from build123d import *

# Parameters (mm, degrees)
SKETCH090_W     = 20
SKETCH090_H     = 10
PAD049_DEPTH    = 10
SKETCH091_W     = 20
SKETCH091_H     = 6
PAD050_DEPTH    = 15
SKETCH092_W     = 1.5
SKETCH092_H     = 15
PAD051_DEPTH    = 0.9
SKETCH093_W     = 17
SKETCH093_H     = 3.5
POCKET033_DEPTH = 16
SKETCH094_W     = 0.8
SKETCH094_H     = 0.3
POCKET034_DEPTH = 20
SKETCH095_W     = 0.8
SKETCH095_H     = 0.3
POCKET035_DEPTH = 20
SKETCH006_W     = 18
SKETCH006_H     = 8
POCKET003_DEPTH = 8
SKETCH096_W     = 0.8
SKETCH096_H     = 0.7
POCKET036_DEPTH = 2
SKETCH097_W     = 0.8
SKETCH097_H     = 0.5
POCKET037_DEPTH = 5
FILLET_R        = 0.17
CHAMFER054_SIZE = 0.3
CHAMFER007_SIZE = 0.3
FILLET001_R     = 0.15


with BuildPart() as part:
    # Sketch090 → Pad049 (new body)
    with BuildSketch(Plane.XZ):
        Rectangle(SKETCH090_W, SKETCH090_H)
    extrude(amount=-PAD049_DEPTH)

    # Sketch091 (on Face5 of Pad049) → Pad050 (join)
    with BuildSketch(Plane.XZ):
        Rectangle(SKETCH091_W, SKETCH091_H)
    extrude(amount=PAD050_DEPTH)

    # Sketch092 (on Face7 of Pad050) → Pad051 (join)
    with BuildSketch(Plane(origin=(0, 0, -3), x_dir=(1, 0, 0), z_dir=(0, 0, -1))):
        with Locations((-7.25, 7.5)):
            Rectangle(SKETCH092_W, SKETCH092_H)
        with Locations((7.25, 7.5)):
            Rectangle(SKETCH092_W, SKETCH092_H)
    extrude(amount=PAD051_DEPTH)

    # Sketch093 (on Face18 of Pad051) → Pocket033 (cut)
    with BuildSketch(Plane.XZ.offset(15)):
        with Locations((0, -0.25)):
            Rectangle(SKETCH093_W, SKETCH093_H)
    extrude(amount=-POCKET033_DEPTH, mode=Mode.SUBTRACT)

    # Sketch094 (on Face9 of Pocket033) → Pocket034 (cut)
    with BuildSketch(Plane.XZ.offset(15)):
        with Locations((-3.4, -2.15)):
            Rectangle(SKETCH094_W, SKETCH094_H)
        with Locations((3.4, -2.15)):
            Rectangle(SKETCH094_W, SKETCH094_H)
    extrude(amount=-POCKET034_DEPTH, mode=Mode.SUBTRACT)

    # Sketch095 (on Face9 of Pocket034) → Pocket035 (cut)
    with BuildSketch(Plane.XZ.offset(15)):
        with Locations((-3.4, -2.85)):
            Rectangle(SKETCH095_W, SKETCH095_H)
        with Locations((3.4, -2.85)):
            Rectangle(SKETCH095_W, SKETCH095_H)
    extrude(amount=-POCKET035_DEPTH, mode=Mode.SUBTRACT)

    # Sketch006 (on Face5 of Pocket035) → Pocket003 (cut)
    with BuildSketch(Plane(origin=(0, 10, 0), x_dir=(1, 0, 0), z_dir=(0, 1, 0))):
        Rectangle(SKETCH006_W, SKETCH006_H)
    extrude(amount=-POCKET003_DEPTH, mode=Mode.SUBTRACT)

    # Sketch096 (on Face21 of Pocket003) → Pocket036 (cut)
    with BuildSketch(Plane(origin=(0, 0, -3), x_dir=(1, 0, 0), z_dir=(0, 0, -1))):
        with Locations((-3.4, 14.65)):
            Rectangle(SKETCH096_W, SKETCH096_H)
        with Locations((3.4, 14.65)):
            Rectangle(SKETCH096_W, SKETCH096_H)
    extrude(amount=-POCKET036_DEPTH, mode=Mode.SUBTRACT)

    # Sketch097 (on Face36 of Pocket036) → Pocket037 (cut)
    with BuildSketch(Plane(origin=(0, 2, 0), x_dir=(1, 0, 0), z_dir=(0, 1, 0))):
        with Locations((-3.4, 2.95)):
            Rectangle(SKETCH097_W, SKETCH097_H)
        with Locations((-3.4, 2.05)):
            Rectangle(SKETCH097_W, SKETCH097_H)
        with Locations((3.4, 2.95)):
            Rectangle(SKETCH097_W, SKETCH097_H)
        with Locations((3.4, 2.05)):
            Rectangle(SKETCH097_W, SKETCH097_H)
    extrude(amount=-POCKET037_DEPTH, mode=Mode.SUBTRACT)

    # Fillet
    fillet_edges = [part.edges().sort_by_distance(p)[0] for p in [
        (-3.4, -14.3, -2.3),
        (-3.4, -14.3, -2.7),
        (3.4, -14.3, -2.3),
        (3.4, -14.3, -2.7),
    ]]
    fillet(fillet_edges, radius=FILLET_R)

    # Chamfer054
    chamfer054_edges = [part.edges().sort_by_distance(p)[0] for p in [
        (-9, -15, -3),
        (-10, -15, 0),
        (0, -15, 3),
        (10, -15, 0),
        (9, -15, -3),
        (8, -15, -3.45),
        (7.25, -15, -3.9),
        (6.5, -15, -3.45),
        (5.15, -15, -3),
        (0, -15, -3),
        (-5.15, -15, -3),
        (-7.25, -15, -3.9),
        (-8, -15, -3.45),
        (-6.5, -15, -3.45),
        (-6.15, -15, -2),
        (0, -15, -2),
        (6.15, -15, -2),
        (8.5, -15, -0.25),
        (0, -15, 1.5),
        (-8.5, -15, -0.25),
        (10, -7.5, 3),
        (10, -7.5, -3),
        (-10, -7.5, -3),
        (-10, -7.5, 3),
        (8, -7.5, -3.9),
        (6.5, -7.5, -3.9),
        (-6.5, -7.5, -3.9),
        (-8, -7.5, -3.9),
    ]]
    chamfer(chamfer054_edges, length=CHAMFER054_SIZE)

    # Chamfer007
    chamfer007_edges = [part.edges().sort_by_distance(p)[0] for p in [
        (0, 10, -4),
        (-9, 10, 0),
        (0, 10, 4),
        (9, 10, 0),
    ]]
    chamfer(chamfer007_edges, length=CHAMFER007_SIZE)

    # Fillet001
    fillet001_edges = [part.edges().sort_by_distance(p)[0] for p in [
        (3.4, 2, -2.3),
        (3.8, 2, -2.05),
        (3.4, 2, -1.8),
        (3, 2, -2.05),
        (3.4, 2, -2.7),
        (3.8, 2, -2.95),
        (3.4, 2, -3.2),
        (3, 2, -2.95),
        (-3.4, 2, -1.8),
        (-3.8, 2, -2.05),
        (-3.4, 2, -2.3),
        (-3, 2, -2.05),
        (-3.4, 2, -2.7),
        (-3.8, 2, -2.95),
        (-3.4, 2, -3.2),
        (-3, 2, -2.95),
    ]]
    fillet(fillet001_edges, radius=FILLET001_R)


with BuildPart() as part_1:
    # Body017 placement: moved
    add(part.part.moved(Location((0, -25, -131.5))))


solid = part_1.part
The listing builds one solid part. Answer for the finished solid, in the listing's coordinates (mm). A direction names the side the tool comes from. Coordinates: 2 decimals unless noted, no trailing zeros. Loops run counter-clockwise (first coordinate to the right, second up) from the corner with the lowest first, then second, coordinate; pieces in that order, holes last. Notation, with made-up numbers: (-21.5, -14) -> (3.5, -14) arc R30 cw to (3.5, 22) -> close; hole circle Ø9 at (71.25, 12.25). An arc over 180 degrees is marked (long way). Answer in a Markdown table with one row per item. Add a question column.
1. Determine the mould class of faces 1 (the flat face through (-10, -25, -132)), 2 (the flat face through (7, -32, -135.4)), 3 (the flat face through (-9, -19, -131)), 4 (the flat face through (0, -20, -126.5)) for opening direction Z: +Z half, -Z half, draft (parallel to the pull), parting line (faces both ways), or undercut.
2. The part is cut by section A-A, the plane x = 3.5. Count the separate pieces of the cut face and the enclosed holes in it, then the cut area to 3 significant figures.
3. The part is cut by section D-D, the plane x = 7.25. Write down the section's boundary in (y, z).
4. The part is cut by section B-B, the plane y = -22.5. Write down the section's boundary in (x, z).
5. For faces 5 (the flat face through (-7, -32, -135.4)), 6 (the flat face through (0, -25, -136)), 7 (the flat face through (0, -23, -132)), 8 (the flat face through (8.5, -32, -132)), determine the directions among +Z, -Z, +X, -X, +Y, -Y from which every point of the face is accessible in a straight line to the end or side of a thin tool.
6. Consider line 1 (X direction, y = -38.5, z = -132); line 2 (Z direction, x = 2, y = -37.5); line 3 (Z direction, x = -6, y = -16). Determine where each line is inside the solid, lowest interval first. Write a range as [from, to].
7. Flat-ended cylindrical pins translate along their axes: P1, Ø4, axis at x = -6, z = -133.5, coming from the -Y side; P2, Ø8, axis at x = -3.5, y = -31, coming from the -Z side; P3, Ø5, axis at x = 0, y = -30.5, coming from the -Z side; P4, Ø4, axis at x = -0.5, y = -28, coming from the +Z side. Find the tip coordinate at first contact, or state that the pin passes through.
8. The part is cut by section C-C, the plane z = -129.25. Write down the section's boundary in (x, y).
Answer below:
| question | item | result |
|---|---|---|
| 1 | face 1 | draft |
| 1 | face 2 | -Z half |
| 1 | face 3 | undercut |
| 1 | face 4 | +Z half |
| 2 | separate pieces | 3 |
| 2 | enclosed holes | 0 |
| 2 | area | 58.7 mm2 |
| 3 | outline | (-40, -135.1) -> (-39.7, -135.4) -> (-25, -135.4) -> (-25, -136.5) -> (-15, -136.5) -> (-15, -135.8) -> (-15.3, -135.5) -> (-23, -135.5) -> (-23, -127.5) -> (-15.3, -127.5) -> (-15, -127.2) -> (-15, -126.5) -> (-25, -126.5) -> (-25, -128.5) -> (-39.7, -128.5) -> (-40, -128.8) -> (-40, -129.7) -> (-39.7, -130) -> (-24, -130) -> (-24, -133.5) -> (-39.7, -133.5) -> (-40, -133.8) -> close |
| 4 | outline | (-10, -136.5) -> (10, -136.5) -> (10, -126.5) -> (-10, -126.5) -> close; hole (-9, -135.5) -> (9, -135.5) -> (9, -127.5) -> (-9, -127.5) -> close |
| 5 | face 5 | -Z, +X, -X, -Y |
| 5 | face 6 | -Z, -Y |
| 5 | face 7 | +Y |
| 5 | face 8 | -Y |
| 6 | line 1 | [-10, -8.5], [8.5, 10] |
| 6 | line 2 | [-134.5, -133.5], [-130, -128.5] |
| 6 | line 3 | [-136.5, -135.5], [-127.5, -126.5] |
| 7 | P1 | y = -40 |
| 7 | P2 | z = -135.4 |
| 7 | P3 | z = -134.5 |
| 7 | P4 | z = -128.5 |
| 8 | outline | (-10, -39.7) -> (-9.7, -40) -> (9.7, -40) -> (10, -39.7) -> (10, -15) -> (9.3, -15) -> (9, -15.3) -> (9, -23) -> (-9, -23) -> (-9, -15.3) -> (-9.3, -15) -> (-10, -15) -> close |
